```python
from build123d import *

# Parameters (mm, degrees)
F0_W     = 76.2
F0_H     = 4.826
F3_DEPTH = 11.176
F4_R     = 4.5085
F5_DEPTH = 50.8


with BuildPart() as f1:
    # F0 (on Front) → F1 (revolve)
    with BuildSketch(Plane.XZ):
        with Locations((-38.1, 2.413)):
            Rectangle(F0_W, F0_H)
        Polygon((0, 4.826), (0, 0), (10.16, 0), (10.16, 10.16), (0, 10.16), align=None)
        with BuildLine():
            Line((10.16, 10.16), (10.16, 0))
            Line((10.16, 0), (18.796, 0))
            Line((18.796, 0), (53.848, 0))
            Line((53.848, 0), (113.792, 0))
            Line((113.792, 0), (113.792, 4.9320105463))
            add(Edge.make_bspline(
                [(10.16, 10.16), (13.7052002053, 11.5489816795), (18.8750721399, 15.575013351), (24.7449167559, 8.7087798176), (38.0188993062, 8.0562980931), (53.997031353, 9.5899815331), (70.7667696282, 14.8120816393), (87.6805073033, 15.3823754953), (105.7530127128, 13.9496938754), (113.0144173366, 8.3257304953), (113.792, 4.9320105463)],
                knots=[0, 0, 0, 0, 0.1043231262, 0.194715736, 0.3169668625, 0.4560481077, 0.598910255, 0.7411190704, 0.8869306816, 1, 1, 1, 1], degree=3))
        make_face()
    revolve(axis=Axis((18.796, 0, 0), (1, 0, 0)))

    # F2 (on Top) → F3 (join)
    with BuildSketch(Plane.XY):
        with BuildLine():
            ThreePointArc((-41.4655, 0), (-44.958, 3.4925), (-48.4505, 0))
            Line((-48.4505, 0), (-41.4655, 0))
        make_face()
        with BuildLine():
            Line((-41.4655, 0), (-48.4505, 0))
            ThreePointArc((-48.4505, 0), (-44.958, -3.4925), (-41.4655, 0))
        make_face()
    extrude(amount=F3_DEPTH)


with BuildPart() as f5:
    # F4 (on face) → F5 (new body)
    with BuildSketch(Plane(origin=(-76.2, 0, 0), x_dir=(0, -1, 0), z_dir=(-1, 0, 0))):
        Circle(F4_R)
    extrude(amount=-F5_DEPTH)


with BuildPart() as f1_1:
    add(f1.part)

    # F6: cut F5
    add(f5.part, mode=Mode.SUBTRACT)


solid = f1_1.part
```
CAD build for the part. Positions are in the model's coordinates, mm. A direction names the side the tool comes from. Give positions to 0.01 mm unless a question says otherwise; leave off trailing zeros. Write each loop counter-clockwise with the first axis right and the second up, starting at its lowest first coordinate (ties: lowest second). Pieces come first, ordered by that corner, then holes. Notation, with made-up numbers: (65.5, 31.5) -> (78.5, 31.5) arc R25 cw to (78.5, 47.5) -> close; hole circle Ø8 at (35.25, 33.5). An arc over 180 degrees is marked (long way). Write each question's results on one line, items separated by ' | '.
1. Wall check: probe 1 along Z at (x, y) = (-50, 0); probe 2 along Z at (x, y) = (-44, 0); probe 3 along Y at (x, z) = (-40.5, 0.5). Give the ranges that are in metal, low to high. Write a range as [from, to].
Geometry check:
probe 1: [-4.83, -4.51], [4.51, 4.83] | probe 2: [-4.83, -4.51], [4.51, 11.18] | probe 3: [-4.8, -4.48], [4.48, 4.8]
2. Drop flat-ended pins along their axis: P1, Ø6, axis at x = -51, y = 2.5, coming from the -Z side; P2, Ø3, axis at x = 27.5, z = 4, coming from the -Y side; P3, Ø4, axis at y = 0, z = -10.5, coming from the +X side. Give the stop position or say it passes through.
Geometry check:
P1: z = -4.83 | P2: y = -9.06 | P3: x = 111.86
3. Which spindle directions (+Z, -Z, +X, -X, +Y, -Y) get a long thin tool onto all of the face, cutting with end or side? Do faces 4 (the cylindrical face through (-51.16, 0.98, -4.4)), 5 (the flat face through (-45, 0, 11.176)), 6 (the cylindrical face through (-42.19, 2.13, 7.2)), 7 (the flat face through (113.792, 0, 0)). Say none if no direction does.
Geometry check:
face 4: -X | face 5: +Z, -X, +Y, -Y | face 6: +Z | face 7: +Z, -Z, +X, +Y, -Y
4. Cut at A-A, the plane x = -59. Write the cut outline in (y, z), then the cut area to 3 significant figures.
Geometry check:
outline: circle Ø9.65 at (0, 0); hole circle Ø9.02 at (0, 0) | area: 9.31 mm²
5. Two-plate mould, pull along Y, no slides. Class faces 1 (the flat face through (-25.4, 0, 0)), 2 (the cylindrical face through (-37.57, -0.21, -4.82)), 3 (the flat face through (0, -2.4, 4.4)): pulls with the +Y half, pulls with the -Y half, needs draft (parallel to the pull), parting line crosses it, or undercut.
Geometry check:
face 1: undercut | face 2: parting line crosses it | face 3: needs draft
